Here's how the part is built. I have some questions about the finished solid (model axes, mm). Face numbers are marked on the shaded views. A direction names the side the tool comes from. Round coordinates to 2 decimals unless told otherwise and drop trailing zeros. Write each loop counter-clockwise with the first axis right and the second up, starting at its lowest first coordinate (ties: lowest second). Pieces come first, ordered by that corner, then holes. Notation, with made-up numbers: (-24.75, 55) -> (23.25, 55) arc R10 ccw to (23.25, 63) -> close; hole circle Ø6 at (6.25, -15.5). An arc over 180 degrees is marked (long way). Answer as CSV lines item,"result".
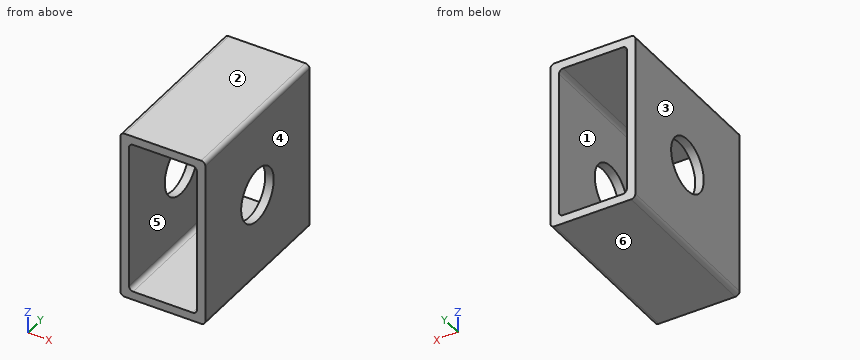
from build123d import *

# Parameters (mm, degrees)
BOSS_EXTRU_1_DEPTH      = 705
ESQUISSE3_R             = 10.125
ESQUISSE3_R_2           = 12.5
ENL_V_MAT_EXTRU_1_DEPTH = 711.651109899
ESQUISSE4_W             = 618.270478043
ESQUISSE4_H             = 899.840554594
ESQUISSE4_W_2           = 40
ESQUISSE4_H_2           = 80
ENL_V_MAT_EXTRU_2_DEPTH = 711.651109899


with BuildPart() as part:
    # Esquisse2 → Boss.-Extru.1 (new body)
    with BuildSketch(Plane(origin=(0, 0, 0), x_dir=(1, 0, 0), z_dir=(0, 1, 0))):
        with BuildLine():
            Line((2, 0), (38, 0))
            ThreePointArc((38, 0), (39.414213562, 0.585786438), (40, 2))
            Line((40, 2), (40, 78))
            ThreePointArc((40, 78), (39.414213562, 79.414213562), (38, 80))
            Line((38, 80), (2, 80))
            ThreePointArc((2, 80), (0.585786438, 79.414213562), (0, 78))
            Line((0, 78), (0, 2))
            ThreePointArc((0, 2), (0.585786438, 0.585786438), (2, 0))
        make_face()
        with BuildLine():
            Line((6, 4), (34, 4))
            ThreePointArc((34, 4), (35.414213562, 4.585786438), (36, 6))
            Line((36, 6), (36, 74))
            ThreePointArc((36, 74), (35.414213562, 75.414213562), (34, 76))
            Line((34, 76), (6, 76))
            ThreePointArc((6, 76), (4.585786438, 75.414213562), (4, 74))
            Line((4, 74), (4, 6))
            ThreePointArc((4, 6), (4.585786438, 4.585786438), (6, 4))
        make_face(mode=Mode.SUBTRACT)
    extrude(amount=BOSS_EXTRU_1_DEPTH)

    # Esquisse3 → Enlèv. mat.-Extru.1 (cut, through all)
    with BuildSketch(Plane(origin=(40, 0, 0), x_dir=(0, 0, -1), z_dir=(1, 0, 0))):
        with Locations((40, 90)):
            Circle(ESQUISSE3_R)
        with Locations((40, 665)):
            Circle(ESQUISSE3_R_2)
    extrude(amount=-ENL_V_MAT_EXTRU_1_DEPTH, mode=Mode.SUBTRACT)

    # Esquisse4 → Enlèv. mat.-Extru.2 (cut, through all)
    with BuildSketch(Plane.XY):
        with Locations((15.340579257, 415.457209906)):
            Rectangle(ESQUISSE4_W, ESQUISSE4_H)
        with Locations((20, 665)):
            Rectangle(ESQUISSE4_W_2, ESQUISSE4_H_2, mode=Mode.SUBTRACT)
    extrude(amount=-ENL_V_MAT_EXTRU_2_DEPTH, mode=Mode.SUBTRACT)


solid = part.part
Item 1: For the marked faces 1 and 2, which set-ups out of +Z, -Z, +X, -X, +Y, -Y let a thin tool reach every point of the face, with its end or its side?
Results found:
face 1,"+Y, -Y"
face 2,"+Z, +X, -X, +Y, -Y"
Item 2: Suppose I cut it at A-A, the plane x = 20.5. List the corners of the cut face in (y, z) for me, then the cut area to 3 significant figures.
Results found:
outline,"(625, -80) -> (705, -80) -> (705, -76) -> (625, -76) -> close; (625, -4) -> (705, -4) -> (705, 0) -> (625, 0) -> close"
area,"640 mm²"
Item 3: I need wall thicknesses on L1, parallel to Z at x = 8, y = 656.5; L2, parallel to X at y = 690, z = -6.5; L3, parallel to Z at x = 2, y = 665. Which ranges of each line are inside material? Lowest first, please.
Results found:
L1,"z = -80 to -76, -4 to 0"
L2,"x = 0 to 4, 36 to 40"
L3,"z = -80 to -52.5, -27.5 to 0"
Item 4: If we mould it in two halves opening along X, with no side actions, what happens to the marked faces 3, 4, 5 and 6? For each: pulls with the +X half, pulls with the -X half, needs draft (parallel to the pull), parting line crosses it, or undercut.
Results found:
face 3,"pulls with the -X half"
face 4,"pulls with the +X half"
face 5,"undercut"
face 6,"needs draft"
Item 5: Suppose I cut it at B-B, the plane y = 636. List the corners of the cut face in (x, z) for me.
Results found:
outline,"(0, -78) arc R2 ccw to (2, -80) -> (38, -80) arc R2 ccw to (40, -78) -> (40, -2) arc R2 ccw to (38, 0) -> (2, 0) arc R2 ccw to (0, -2) -> close; hole (4, -74) arc R2 ccw to (6, -76) -> (34, -76) arc R2 ccw to (36, -74) -> (36, -6) arc R2 ccw to (34, -4) -> (6, -4) arc R2 ccw to (4, -6) -> close"
Item 6: Suppose I cut it at C-C, the plane z = -40. List the corners of the cut face in (x, y) for me, then the cut area to 3 significant figures.
Results found:
outline,"(0, 625) -> (4, 625) -> (4, 652.5) -> (0, 652.5) -> close; (0, 677.5) -> (4, 677.5) -> (4, 705) -> (0, 705) -> close; (36, 625) -> (40, 625) -> (40, 652.5) -> (36, 652.5) -> close; (36, 677.5) -> (40, 677.5) -> (40, 705) -> (36, 705) -> close"
area,"440 mm²"
Item 7: Suppose I cut it at D-D, the plane y = 665. List the corners of the cut face in (x, z) for me, then the cut area to 3 significant figures.
Results found:
outline,"(0, -78) arc R2 ccw to (2, -80) -> (38, -80) arc R2 ccw to (40, -78) -> (40, -52.5) -> (36, -52.5) -> (36, -74) arc R2 cw to (34, -76) -> (6, -76) arc R2 cw to (4, -74) -> (4, -52.5) -> (0, -52.5) -> close; (0, -27.5) -> (4, -27.5) -> (4, -6) arc R2 cw to (6, -4) -> (34, -4) arc R2 cw to (36, -6) -> (36, -27.5) -> (40, -27.5) -> (40, -2) arc R2 ccw to (38, 0) -> (2, 0) arc R2 ccw to (0, -2) -> close"
area,"696 mm²"
